Can you work these out from the model? Positions are in its coordinate system, mm. A direction names the side the tool comes from. Round coordinates to 2 decimals unless told otherwise and drop trailing zeros. Write each loop counter-clockwise with the first axis right and the second up, starting at its lowest first coordinate (ties: lowest second). Pieces come first, ordered by that corner, then holes. Notation, with made-up numbers: (22, -10) - (52, -10) arc R18 cw to (52, 19) - close; hole circle Ø4 at (28, 59). An arc over 180 degrees is marked (long way). One line per item, written item: value. Start each with the question number.
(1) I want a section at C-C on x = 154. List the corners of the cut face in (y, z) for me.
(2) Thinking about a two-plate mould opening in Z: for faces 5 (the face through (0, 1, 0)), 6 (the face through (146.667, 1, 20)), 7 (the face through (54, 1, -18.5)), which applies, +Z half, -Z half, draft (parallel to the pull), parting line (faces both ways), or undercut?
(3) I'm going to push flat-ended pins straight in: pin 1 Ø4 at (x, z) = (158, 10.5) entering from +Y (3 decimals); pin 2 Ø0.9 at (x, y) = (117.5, 2) entering from +Z; pin 3 Ø1.5 at (y, z) = (1, -20.5) entering from -X. Where does each tip first touch, or does it pass through?
(4) If I drill on L1, parallel to Z at x = 143, y = 2.7; L2, parallel to Z at x = 91.5, y = 2.3; L3, parallel to X at y = 2.1, z = 10.5, over which ranges is the centre line in solid material (lowest first)? Write a range as from..to.
(5) I want a section at A-A on x = 23. List the corners of the cut face in (y, z) for me.
(6) On a 3-axis mill with a long thin cutter (end or side, diameter ignored), from which of +Z, -Z, +X, -X, +Y, -Y can I reach the whole of each face in a straight line? I mean faces 1 (the face through (106.667, 1, 20)), 2 (the face through (-2, 1, 18.5)), 3 (the face through (-2, 1, -18.5)), 4 (the face through (146.667, 1, -20)). Say none if no direction works.
(7) I want a section at D-D on y = 2.1. Give the number of separate pieces and of enclosed holes in the cut face, plus the area to 3 significant figures.
(8) I want a section at B-B on z = -7. List the corners of the cut face in (x, y) for me.
from build123d import *

# Parameters (mm, degrees)
SKETCH1_W           = 3
SKETCH1_H           = 19
SKETCH1_R           = 1
SKETCH1_R_2         = 13.5
BOSS_EXTRUDE1_DEPTH = 3


with BuildPart() as part:
    # Sketch1 → Boss-Extrude1 (new body)
    with BuildSketch(Plane(origin=(0, 0, 0), x_dir=(1, 0, 0), z_dir=(0, 1, 0))):
        Polygon((33.333333333, 21.5), (0, 21.5), (0, 18.5), (-4, 18.5), (-4, -18.5), (0, -18.5), (0, -21.5), (33.333333333, -21.5), (33.333333333, -18.5), (73.333333333, -18.5), (73.333333333, -21.5), (106.666666667, -21.5), (106.666666667, -18.5), (146.666666667, -18.5), (146.666666667, -21.5), (180, -21.5), (180, 21.5), (146.666666667, 21.5), (146.666666667, 18.5), (106.666666667, 18.5), (106.666666667, 21.5), (73.333333333, 21.5), (73.333333333, 18.5), (33.333333333, 18.5), align=None)
        with Locations((1.5, 0)):
            Rectangle(SKETCH1_W, SKETCH1_H, mode=Mode.SUBTRACT)
        with Locations((74.375, -13)):
            Circle(SKETCH1_R, mode=Mode.SUBTRACT)
        with Locations((142.875, -13)):
            Circle(SKETCH1_R, mode=Mode.SUBTRACT)
        with Locations((23, 0)):
            Circle(SKETCH1_R_2, mode=Mode.SUBTRACT)
        with Locations((57.25, 0)):
            Circle(SKETCH1_R_2, mode=Mode.SUBTRACT)
        with Locations((74.375, 13)):
            Circle(SKETCH1_R, mode=Mode.SUBTRACT)
        with Locations((91.5, 0)):
            Circle(SKETCH1_R_2, mode=Mode.SUBTRACT)
        with Locations((125.75, 0)):
            Circle(SKETCH1_R_2, mode=Mode.SUBTRACT)
        with Locations((160, 0)):
            Circle(SKETCH1_R_2, mode=Mode.SUBTRACT)
        with Locations((142.875, 13)):
            Circle(SKETCH1_R, mode=Mode.SUBTRACT)
    extrude(amount=BOSS_EXTRUDE1_DEPTH)


solid = part.part
Established:
1. outline: (0, -21.5) - (3, -21.5) - (3, -12.09) - (0, -12.09) - close; (0, 12.09) - (3, 12.09) - (3, 21.5) - (0, 21.5) - close
2. face 5: undercut
2. face 6: draft
2. face 7: -Z half
3. pin 1: through
3. pin 2: z = 18.5
3. pin 3: x = 0
4. L1: -18.5..-13.99, -12.01..12.01, 13.99..18.5
4. L2: -21.5..-13.5, 13.5..21.5
4. L3: -4..14.51, 31.49..48.76, 65.74..83.01, 99.99..117.26, 134.24..151.51, 168.49..180
5. outline: (0, -21.5) - (3, -21.5) - (3, -13.5) - (0, -13.5) - close; (0, 13.5) - (3, 13.5) - (3, 21.5) - (0, 21.5) - close
6. face 1: +Z, +Y, -Y
6. face 2: +Z, -X, +Y, -Y
6. face 3: -Z, -X, +Y, -Y
6. face 4: -Z, +Y, -Y
7. separate pieces: 1
7. enclosed holes: 10
7. area: 4,480 mm2
8. outline: (-4, 0) - (0, 0) - (0, 3) - (-4, 3) - close; (3, 0) - (11.46, 0) - (11.46, 3) - (3, 3) - close; (34.54, 0) - (45.71, 0) - (45.71, 3) - (34.54, 3) - close; (68.79, 0) - (79.96, 0) - (79.96, 3) - (68.79, 3) - close; (103.04, 0) - (114.21, 0) - (114.21, 3) - (103.04, 3) - close; (137.29, 0) - (148.46, 0) - (148.46, 3) - (137.29, 3) - close; (171.54, 0) - (180, 0) - (180, 3) - (171.54, 3) - close
